```python
from build123d import *

# Parameters (mm, degrees)
F1_R     = 2.75
F1_R_2   = 1.5
F2_DEPTH = 2
F3_START = 1.5
F3_DEPTH = 0.5
F4_START = 2
F4_DEPTH = 11
F5_SIZE2 = 1.25
F5_SIZE  = 1.25
F6_R     = 0.25


# Not quite as in the source:
# - a feature names something its author has since deleted; it is built from what else it names


with BuildPart() as f2:
    # F1 (on Top) → F2 (new body)
    with BuildSketch(Plane.XY):
        Circle(F1_R)
        Circle(F1_R_2, mode=Mode.SUBTRACT)
        Circle(F1_R_2)
        Polygon((-0.5773502692, -1), (-1.1547005384, 0), (-0.5773502692, 1), (0.5773502692, 1), (1.1547005384, 0), (0.5773502692, -1), align=None, mode=Mode.SUBTRACT)
    extrude(amount=F2_DEPTH)

    # F1 (on Top) → F3 (join)
    with BuildSketch(Plane.XY.offset(F3_START)):
        Polygon((-0.5773502692, 1), (-1.1547005384, 0), (-0.5773502692, -1), (0.5773502692, -1), (1.1547005384, 0), (0.5773502692, 1), align=None)
    extrude(amount=F3_DEPTH)

    # F1 (on Top) → F4 (join)
    with BuildSketch(Plane.XY.offset(F4_START)):
        Circle(F1_R_2)
        Polygon((-0.5773502692, -1), (-1.1547005384, 0), (-0.5773502692, 1), (0.5773502692, 1), (1.1547005384, 0), (0.5773502692, -1), align=None, mode=Mode.SUBTRACT)
        Polygon((-0.5773502692, 1), (-1.1547005384, 0), (-0.5773502692, -1), (0.5773502692, -1), (1.1547005384, 0), (0.5773502692, 1), align=None)
    extrude(amount=F4_DEPTH)

    # F5
    f5_edges = [f2.edges().sort_by_distance(p)[0] for p in [
        (-2.75, 0, 0),
    ]]
    chamfer(f5_edges, length=F5_SIZE, length2=F5_SIZE2)

    # F6
    f6_edges = [f2.edges().sort_by_distance(p)[0] for p in [
        (-2.75, 0, 2),
        (-1.5, 0, 2),
        (-1.5, 0, 0),
        (-2.75, 0, 1.25),
    ]]
    fillet(f6_edges, radius=F6_R)


solid = f2.part
```
For this review, take the finished solid that the model builds, in its own axes (mm). A direction names the side the tool comes from. Round coordinates to 2 decimals unless told otherwise and drop trailing zeros. Write each loop counter-clockwise with the first axis right and the second up, starting at its lowest first coordinate (ties: lowest second). Pieces come first, ordered by that corner, then holes.
1) Insertion check: pin 1 Ø1 at (y, z) = (-1.5, 8.5) entering from +X; pin 2 Ø0.6 at (x, z) = (0, 1) entering from -Y; pin 3 Ø2 at (x, z) = (0.5, 6.5) entering from -Y. Each pin has a flat end and moves straight along its axis. Give the tip position at first contact, or say it passes through.
Answer below:
pin 1: stops at x = 1.12
pin 2: stops at y = -2.74
pin 3: stops at y = -1.5
2) For line 1 along Y through (x, z) = (-0.55, 0.5); line 2 along X through (y, z) = (0.9, 3.75); line 3 along X through (y, z) = (-0.05, 3), list the stretches that pass through material, from the lowest coordinate up.
Answer below:
line 1: y = -1.92 to -1, 1 to 1.92
line 2: x = -1.2 to 1.2
line 3: x = -1.5 to 1.5
3) Machinability: for faces 1 (the face through (-0.86, -0.51, 0.74)), 2 (the face through (0, 0, 13)), which of the approach directions +Z, -Z, +X, -X, +Y, -Y give a long, thin tool a straight path to every point of the face, cutting with its end or side? Answer none if there is none.
Answer below:
face 1: -Z
face 2: +Z, +X, -X, +Y, -Y
4) Take a section at A-A on z = 12. Give the boundary of the cut face in (x, y).
Answer below:
outline: circle Ø3 at (0, 0)
5) Mouldability with a two-part tool opening along Y and no side actions: class faces 3 (the face through (1, 2, 2)), 4 (the face through (0, -1, 1)), 5 (the face through (-1.5, 0.07, 7.55)) as +Y half, -Y half, draft (parallel to the pull), parting line (faces both ways), or undercut.
Answer below:
face 3: draft
face 4: undercut
face 5: parting line
